from build123d import *

# Parameters (mm, degrees)
SKETCH1_R           = 90
SKETCH1_R_2         = 5
SKETCH1_R_3         = 60
BOSS_EXTRUDE1_DEPTH = 5
SKETCH2_R           = 60
BOSS_EXTRUDE2_DEPTH = 5
DOME1_FACE_RADIUS   = 60
DOME1_HEIGHT        = 20
BOSS_EXTRUDE3_START = 5
SKETCH3_R           = 60
BOSS_EXTRUDE3_DEPTH = 5
FILLET2_R           = 2.5


with BuildPart() as part:
    # Sketch1 → Boss-Extrude1 (new body)
    with BuildSketch(Plane(origin=(0, 0, 0), x_dir=(0, 0, -1), z_dir=(1, 0, 0))):
        Circle(SKETCH1_R)
        with Locations((0, 75)):
            Circle(SKETCH1_R_2, mode=Mode.SUBTRACT)
        with Locations((25.651571057, 70.477288579)):
            Circle(SKETCH1_R_2, mode=Mode.SUBTRACT)
        with Locations((48.209304682, 57.453976022)):
            Circle(SKETCH1_R_2, mode=Mode.SUBTRACT)
        with Locations((64.952405284, 37.500866025)):
            Circle(SKETCH1_R_2, mode=Mode.SUBTRACT)
        with Locations((73.861407828, 13.024598133)):
            Circle(SKETCH1_R_2, mode=Mode.SUBTRACT)
        with Locations((73.861755124, -13.022628517)):
            Circle(SKETCH1_R_2, mode=Mode.SUBTRACT)
        with Locations((64.953405284, -37.499133975)):
            Circle(SKETCH1_R_2, mode=Mode.SUBTRACT)
        with Locations((48.210836771, -57.452690446)):
            Circle(SKETCH1_R_2, mode=Mode.SUBTRACT)
        with Locations((25.653450442, -70.476604539)):
            Circle(SKETCH1_R_2, mode=Mode.SUBTRACT)
        with Locations((0.002, -75)):
            Circle(SKETCH1_R_2, mode=Mode.SUBTRACT)
        with Locations((-25.649571057, -70.477288579)):
            Circle(SKETCH1_R_2, mode=Mode.SUBTRACT)
        with Locations((-48.207304682, -57.453976022)):
            Circle(SKETCH1_R_2, mode=Mode.SUBTRACT)
        with Locations((-64.950405284, -37.500866025)):
            Circle(SKETCH1_R_2, mode=Mode.SUBTRACT)
        with Locations((-73.859407828, -13.024598133)):
            Circle(SKETCH1_R_2, mode=Mode.SUBTRACT)
        with Locations((-73.859755124, 13.022628517)):
            Circle(SKETCH1_R_2, mode=Mode.SUBTRACT)
        with Locations((-64.951405284, 37.499133975)):
            Circle(SKETCH1_R_2, mode=Mode.SUBTRACT)
        with Locations((-48.208836771, 57.452690446)):
            Circle(SKETCH1_R_2, mode=Mode.SUBTRACT)
        with Locations((-25.651450442, 70.476604539)):
            Circle(SKETCH1_R_2, mode=Mode.SUBTRACT)
        Circle(SKETCH1_R_3, mode=Mode.SUBTRACT)
    extrude(amount=BOSS_EXTRUDE1_DEPTH)



with BuildPart() as body_2:
    # Sketch2 → Boss-Extrude2 (new body)
    with BuildSketch(Plane(origin=(5, 0, 0), x_dir=(0, 0, -1), z_dir=(1, 0, 0))):
        Circle(SKETCH2_R)
    extrude(amount=BOSS_EXTRUDE2_DEPTH)

    # Dome1: a dome of height H over a round flat face of radius A is a cap of a sphere of radius (A * A + H * H) / (2 * H)
    dome1_r = (DOME1_FACE_RADIUS * DOME1_FACE_RADIUS + DOME1_HEIGHT * DOME1_HEIGHT) / (2 * DOME1_HEIGHT)
    dome1_base = Plane((10, 0, 0), z_dir=(1, 0, 0))
    with Locations(dome1_base.offset(DOME1_HEIGHT - dome1_r)):
        dome1_ball = Sphere(dome1_r, mode=Mode.PRIVATE)
    add(split(dome1_ball, bisect_by=dome1_base, keep=Keep.TOP, mode=Mode.PRIVATE))


with BuildPart() as part_1:
    add(part.part)

    add(body_2.part)  # Boss-Extrude3 merges body 2
    # Sketch3 → Boss-Extrude3 (add)
    with BuildSketch(Plane.ZY.offset(-5).offset(BOSS_EXTRUDE3_START)):
        with Locations(Location((0, 0, 0), (0, 0, 180))):
            Circle(SKETCH3_R)
    extrude(amount=-BOSS_EXTRUDE3_DEPTH)

    # Fillet2
    fillet2_edges = [part_1.edges().sort_by_distance(p)[0] for p in [
        (5, 0, 60),
        (10, -60, 0),
    ]]
    fillet(fillet2_edges, radius=FILLET2_R)


solid = part_1.part
Can you work these out from the model? Positions are in its coordinate system, mm. A direction names the side the tool comes from. Coordinates: 2 decimals unless noted, no trailing zeros. Order: outer loops, then holes, each group sorted by start corner. A loop starts at its lowest first (then second) coordinate and runs counter-clockwise, first axis right, second up. Notation, with made-up numbers: (77, -11.75) - (119, -11.75) arc R8 cw to (119, -0.75) - close; hole circle Ø4 at (24, -17.5). An arc over 180 degrees is marked (long way). Answer as a JSON object with one key per item and string values. Group by question number.
Q1. On a 3-axis mill with a long thin cutter (end or side, diameter ignored), from which of +Z, -Z, +X, -X, +Y, -Y can I reach the whole of each face in a straight line? I mean faces 4 (the face through (2.46, 14.52, 69.09)), 5 (the face through (8.11, 2.64, 59.94)). Say none if no direction works.
Q2. We'd pull the mould along Y, two halves only. Please class faces 1 (the face through (2.465, 65.596, 26.735)), 2 (the face through (2.465, -79.845, -41.53)), 3 (the face through (0, -1, 1)): +Y half, -Y half, draft (parallel to the pull), parting line (faces both ways), or undercut.
Q3. Imagine slicing it at A-A (y = -40). Give the number of separate pieces and of enclosed holes in the cut face, and give its area (3 significant figures).
Q4. I need wall thicknesses on line 1 (Y direction, x = 3.25, z = 23.5); line 2 (X direction, y = 69, z = -3); line 3 (X direction, y = -61, z = -10.5). Which ranges of each line are inside material? Lowest first, please. Write a range as from..to.
Q5. Imagine slicing it at B-B (x = 24.75). Please give me the cut outline in (y, z).
Q6. Will these pins go through, and if not, where does the flat tip stop? P1, Ø16, axis at y = -37.5, z = 64.95, coming from the +X side; P2, Ø2, axis at x = 11.5, z = 42.5, coming from the -Y side; P3, Ø8, axis at y = -75, z = -0.002, coming from the -X side; P4, Ø5, axis at y = 58, z = 4.5, coming from the +X side.
Determined:
{
 "1": {"face 4": "+X, -X", "face 5": "+X"},
 "2": {"face 1": "undercut", "face 2": "parting line", "face 3": "draft"},
 "3": {"separate pieces": "3", "enclosed holes": "0", "area": "1,870 mm2"},
 "4": {"line 1": "y = -86.88..-74.99, -65.96..65.96, 74.99..86.88", "line 2": "x = 0..5", "line 3": "x = 0..5.07"},
 "5": {"outline": "circle Ø63.95 at (0, 0)"},
 "6": {"P1": "stops at x = 5", "P2": "stops at y = -41.62", "P3": "passes through", "P4": "stops at x = 13.07"}
}
